```python
from build123d import *

# Parameters (mm, degrees)
SKETCH_2_W          = 2
SKETCH_2_H          = 3.593987872
SKETCH_2_H_2        = 6.667892238
CUT_EXTRUDE_1_DEPTH = 39.5


with BuildPart() as part:
    # 草图1 → 旋转1 (revolve)
    with BuildSketch(Plane.XY, mode=Mode.PRIVATE) as revolve_1_sk:
        Polygon((-12.25, 12), (-14.25, 12), (-14.25, 8), (-13.75, 8), (-13.75, 7), (-25.4, 7), (-25.4, 5), (-23.5, 5), (-23.5, 4), (-24, 4), (-24, 0), (-20.5, 0), (-20.5, 4), (-21.1, 4), (-21.1, 5), (-12.25, 5), align=None)
    revolve(revolve_1_sk.sketch.rotate(Axis((0, 22.677499451, 0), (0, -1, 0)), 270), axis=Axis((0, 22.677499451, 0), (0, -1, 0)))  # turned: the seam where the file's is

    # 草图2 → 切除-拉伸1 (cut, symmetric)
    with BuildSketch(Plane(origin=(0, 0, 0), x_dir=(0, 0, -1), z_dir=(1, 0, 0))):
        with Locations((0, 11.796993936)):
            Rectangle(SKETCH_2_W, SKETCH_2_H)
        with Locations((0, -1.333946119)):
            Rectangle(SKETCH_2_W, SKETCH_2_H_2)
    extrude(amount=CUT_EXTRUDE_1_DEPTH, both=True, mode=Mode.SUBTRACT)


solid = part.part
```
Geometry: final body of the model. Coordinates: model frame, mm. A direction names the side the tool comes from. Give positions to 0.01 mm unless a question says otherwise; leave off trailing zeros. Loops run counter-clockwise (first coordinate to the right, second up) from the corner with the lowest first, then second, coordinate; pieces in that order, holes last. Notation, with made-up numbers: (39, 51) -> (53, 51) arc R30 ccw to (53, 90) -> close; hole circle Ø2 at (10.5, 68). An arc over 180 degrees is marked (long way). Return JSON: item names as keys, results as strings.
Item 1: Pin query (flat end, axial travel): P1, Ø1.5, axis at x = -9, z = 8.5, coming from the -Y side; P2, Ø1.6, axis at x = -12.5, y = 11.5, coming from the +Z side; P3, Ø4, axis at x = -10.5, y = 6.5, coming from the +Z side. Return the tip coordinate at first contact, or that it passes through.
Filled in:
{"P1": "y = 5", "P2": "z = 8.13", "P3": "z = 23.94"}
Item 2: Access query for faces 1 (the flat face through (22.5, 5, 7.4)), 2 (the flat face through (-13, 10, 0)), 3 (the flat face through (22, 1, 1)). Directions: +Z, -Z, +X, -X, +Y, -Y. A direction counts if a zero-diameter tool reaches every point of the face in a straight line with its end or side. Return the directions, or none.
Filled in:
{"face 1": "none", "face 2": "+X, -X, +Y", "face 3": "+X, -X, -Y"}
Item 3: Line query: line 1 (X direction, y = 4.25, z = 0); line 2 (Y direction, x = 3, z = 21); line 3 (Y direction, x = 6, z = 12.5). Output: solid intervals per line, ascending.
Filled in:
{"line 1": "-23.5 to -21.1, 21.1 to 23.5", "line 2": "0 to 7", "line 3": "5 to 7, 8 to 12"}
Item 4: Section D-D, the plane x = 15. Output: boundary loops of the cut face in (y, z) (3 decimals), plus the area to 3 significant figures.
Filled in:
{"outline": "(0, -18.735) -> (4, -18.735) -> (4, -18.09) -> (5, -18.09) -> (5, -20.498) -> (7, -20.498) -> (7, 20.498) -> (5, 20.498) -> (5, 18.09) -> (4, 18.09) -> (4, 18.735) -> (0, 18.735) -> (0, 13.973) -> (4, 13.973) -> (4, 14.839) -> (5, 14.839) -> (5, -14.839) -> (4, -14.839) -> (4, -13.973) -> (0, -13.973) -> close", "area": "127 mm^2"}
Item 5: Mould query, pull axis Y, two halves, no side actions, for faces 4 (the flat face through (-5, 8, -13)), 5 (the flat face through (13, 11, 1)), 6 (the flat face through (2, 0, 21)), 7 (the flat face through (-20.42, 4, 3.22)). Classes: released by +Y, released by -Y, zero draft, split by the parting line, or undercut.
Filled in:
{"face 4": "undercut", "face 5": "zero draft", "face 6": "released by -Y", "face 7": "undercut"}
